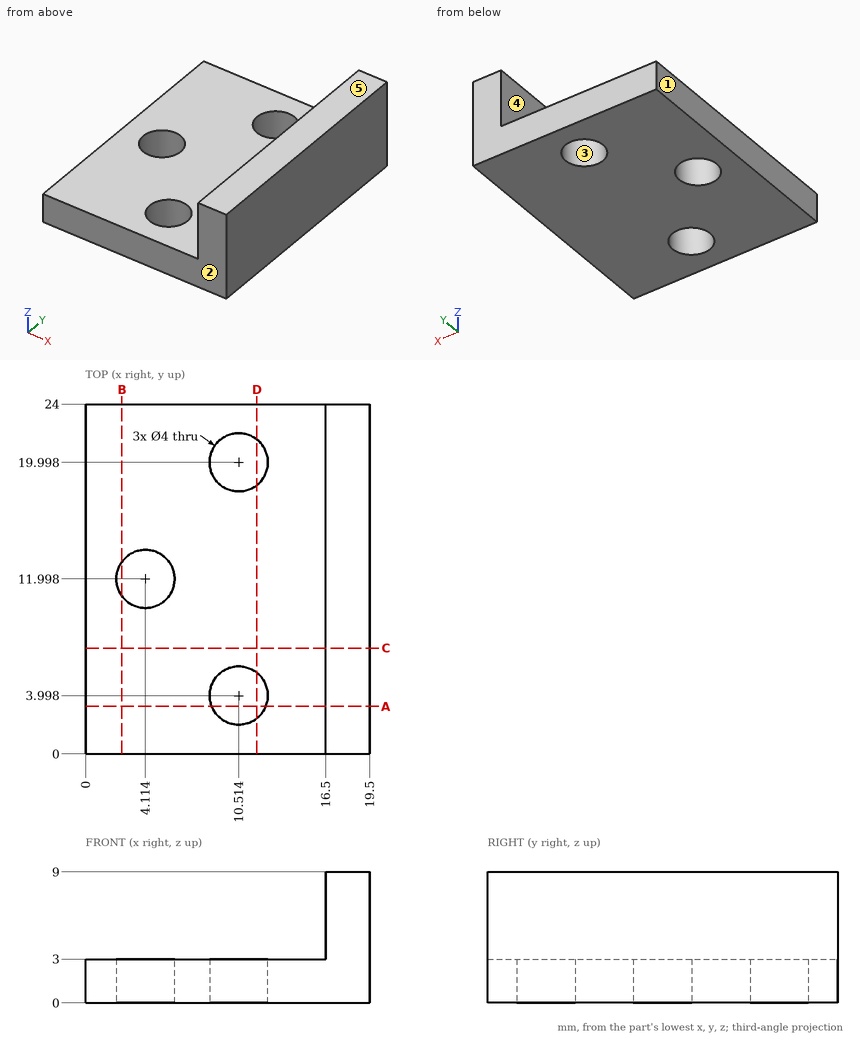
Check sheet for the drawn part. Datum: minimum x, y, z corner. Units: mm. A direction names the side the tool comes from. Give positions to 0.01 mm unless a question says otherwise; leave off trailing zeros. Loops run counter-clockwise (first coordinate to the right, second up) from the corner with the lowest first, then second, coordinate; pieces in that order, holes last. Notation, with made-up numbers: M 4,-1.5 L 45,-1.5 A4 cw 45,4.5 Z; hole C -36.5,34 d7. An arc over 180 degrees is marked long. Answer as CSV lines item,"result".
Item 1: Draft check along X on the marked faces 1, 2 and 3. Enter one of: pulls with the +X half, pulls with the -X half, needs draft (parallel to the pull), parting line crosses it, or undercut.
Reply:
face 1,"pulls with the -X half"
face 2,"needs draft"
face 3,"undercut"
Item 2: Depth check by flat-ended pin: pin 1 Ø6.5 at (x, y) = (4.11, 12) entering from +Z; pin 2 Ø3 at (y, z) = (8, 6.5) entering from -X. Enter the tip coordinate at first touch or a pass-through.
Reply:
pin 1,"z = 3"
pin 2,"x = 16.5"
Item 3: Sectioned sample at C-C, the plane y = 7.25. Enter the section's corners in (x, z), then the cut area to 3 significant figures.
Reply:
outline,"M 0,0 L 19.5,0 L 19.5,9 L 16.5,9 L 16.5,3 L 0,3 Z"
area,"76.5 mm^2"
Item 4: Sectioned sample at D-D, the plane x = 11.75. Enter the section's corners in (y, z).
Reply:
outline,"M 0,0 L 2.43,0 L 2.43,3 L 0,3 Z; M 5.57,0 L 18.43,0 L 18.43,3 L 5.57,3 Z; M 21.57,0 L 24,0 L 24,3 L 21.57,3 Z"
Item 5: Sectioned sample at B-B, the plane x = 2.5. Enter the section's corners in (y, z), then the cut area to 3 significant figures.
Reply:
outline,"M 0,0 L 10.82,0 L 10.82,3 L 0,3 Z; M 13.18,0 L 24,0 L 24,3 L 13.18,3 Z"
area,"64.9 mm^2"
Item 6: Set-up check for the marked faces 4 and 5: record each of +Z, -Z, +X, -X, +Y, -Y from which the full face is reachable in a straight line by a thin tool's end or side.
Reply:
face 4,"+Z, -X, +Y, -Y"
face 5,"+Z, +X, -X, +Y, -Y"
Item 7: Sectioned sample at A-A, the plane y = 3.25. Enter the section's corners in (x, z).
Reply:
outline,"M 0,0 L 8.66,0 L 8.66,3 L 0,3 Z; M 12.37,0 L 19.5,0 L 19.5,9 L 16.5,9 L 16.5,3 L 12.37,3 Z"
Item 8: Scan lines: L1, parallel to Z at x = 3, y = 23; L2, parallel to X at y = 1.75, z = 3.5; L3, parallel to X at y = 5.5, z = 2.75 (1 decimal). Record each from-to range of solid material in increasing order.
Reply:
L1,"0 to 3"
L2,"16.5 to 19.5"
L3,"0 to 9.2, 11.8 to 19.5"
